Autodesk Inventor part; units mm, degrees
ref_plane "作業平面1" through (-6, -360, -20) normal (0, 0, -1) x (0, 1, 0)
ref_plane "YZ Plane" through (0, 0, 0) normal (1, 0, 0) x (0, 1, 0)
ref_plane "XZ Plane" through (0, 0, 0) normal (0, 1, 0) x (-1, 0, 0)
sketch "スケッチ1" plane through (0, 0, 0) normal (0, 0, 1) x (1, 0, 0)
  line L0 (0, 0) -> (-100, 0)
  line L1 (-100, 0) -> (-100, -360)
  line L2 (-100, -360) -> (0, -360)
  line L3 (0, -360) -> (0, 0)
  dimension "d0" = 100
  dimension "d1" = 360
ref_plane "作業平面1" through (-6, -360, -20) normal (0, 0, -1) x (0, 1, 0)
extrude "押し出し1" add sketch "スケッチ1" against normal up to surface (20 mm away)
sketch "スケッチ3" plane through (0, 0, 0) normal (0, 0, 1) x (1, 0, 0)
  line L0 (0, -360) -> (0, 0)
  line L1 (0, 0) -> (-100, 0)
  line L2 (-100, 0) -> (-100, -360)
  line L3 (-100, -360) -> (0, -360)
  line L4 (-5, -5) -> (-95, -5)
  line L5 (-95, -5) -> (-95, -360)
  line L6 (-95, -360) -> (-5, -360)
  line L7 (-5, -360) -> (-5, -5)
  point P0 (-5, -360)
  dimension "d4" = 5
  dimension "d5" = 5
  dimension "d6" = 5
  dimension "d7" = 0
extrude "押し出し2" cut sketch "スケッチ3" against normal up to surface (20 mm away) contours L3 L5 L4 L7
properties part number "arm1"
The model under review builds one solid part; all positions refer to its coordinate system, in mm. A direction names the side the tool comes from. Give positions to 0.01 mm unless a question says otherwise; leave off trailing zeros. Write each loop counter-clockwise with the first axis right and the second up, starting at its lowest first coordinate (ties: lowest second). Pieces come first, ordered by that corner, then holes. Notation, with made-up numbers: M -25.75,10.5 L -7.75,10.5 A11 cw -7.75,26.5 Z; hole C 35,-3.5 d3. An arc over 180 degrees is marked long. Answer in a Markdown table with one row per item.
Item 1: For P1, Ø10, axis at y = -252.5, z = -12, coming from the +X side; P2, Ø3, axis at x = -36.5, z = -5.5, coming from the -Y side, all flat-tipped, find the tip position at first contact; note any pin that passes through.
Check sheet entries:
| item | result |
|---|---|
| P1 | x = 0 |
| P2 | y = -5 |
Item 2: For line 1 along X through (y, z) = (-36.5, -4.5); line 2 along Y through (x, z) = (-80.5, -18.25), list the stretches that pass through material, from the lowest coordinate up.
Check sheet entries:
| item | result |
|---|---|
| line 1 | -100 to -95, -5 to 0 |
| line 2 | -5 to 0 |
Item 3: Add section C-C on x = -84.5. Give the boundary of the cut face in (y, z), plus the area to 3 significant figures.
Check sheet entries:
| item | result |
|---|---|
| outline | M -5,-20 L 0,-20 L 0,0 L -5,0 Z |
| area | 100 mm2 |
Item 4: Tool access review of faces 4 (the face through (-100, -177, -10)), 5 (the face through (-95, -180, -10)): name each direction out of +Z, -Z, +X, -X, +Y, -Y from which nothing blocks a thin tool from reaching the whole face with its end or side.
Check sheet entries:
| item | result |
|---|---|
| face 4 | +Z, -Z, -X, +Y, -Y |
| face 5 | +Z, -Z, -Y |
Item 5: Draft analysis for pull direction X (two halves, no side actions). For faces 1 (the face through (0, -183, -10)), 2 (the face through (-49, -5, -10)), 3 (the face through (-98, -179, 0)), state which applies: +X half, -X half, draft (parallel to the pull), parting line (faces both ways), or undercut.
Check sheet entries:
| item | result |
|---|---|
| face 1 | +X half |
| face 2 | undercut |
| face 3 | draft |
Item 6: Add section A-A on y = -132. Give the boundary of the cut face in (x, z), plus the area to 3 significant figures.
Check sheet entries:
| item | result |
|---|---|
| outline | M -100,-20 L -95,-20 L -95,0 L -100,0 Z; M -5,-20 L 0,-20 L 0,0 L -5,0 Z |
| area | 200 mm2 |
Item 7: Add section B-B on z = -10.75. Give the boundary of the cut face in (x, y).
Check sheet entries:
| item | result |
|---|---|
| outline | M -100,-360 L -95,-360 L -95,-5 L -5,-5 L -5,-360 L 0,-360 L 0,0 L -100,0 Z |
